from build123d import *

# Parameters (mm, degrees)
SKETCH_1_R          = 13
SKETCH_1_R_2        = 4
SKETCH_1_R_3        = 1.6
SKETCH_1_W          = 26
SKETCH_1_H          = 3
EXTRUDE_1_DEPTH     = 3
SKETCH_2_W          = 26
SKETCH_2_H          = 3
EXTRUDE_2_DEPTH     = 28
SKETCH_3_R          = 5
SKETCH_3_R_2        = 2
CUT_EXTRUDE_1_DEPTH = 44.0464865
EXTRUDE_3_DEPTH     = 3


with BuildPart() as part:
    # Sketch 1 → Extrude 1 (new body)
    # profile 1 of 3: a face of its own
    with BuildSketch(Plane(origin=(0, 0, 0), x_dir=(1, 0, 0), z_dir=(0, 1, 0))):
        Circle(SKETCH_1_R)
        with Locations(Location((0, 0, 0), (0, 0, 270))):
            Circle(SKETCH_1_R_2, mode=Mode.SUBTRACT)
        with Locations(Location((-8.5, 0, 0), (0, 0, 270))):
            Circle(SKETCH_1_R_3, mode=Mode.SUBTRACT)
        with Locations(Location((8.5, 0, 0), (0, 0, 270))):
            Circle(SKETCH_1_R_3, mode=Mode.SUBTRACT)
    # profile 2 of 3: a face of its own
    with BuildSketch(Plane(origin=(0, 0, 0), x_dir=(1, 0, 0), z_dir=(0, 1, 0))):
        with BuildLine():
            ThreePointArc((13, 0), (0, -13), (-13, 0))
            Line((-13, 0), (-13, -17))
            Line((-13, -17), (13, -17))
            Line((13, -17), (13, 0))
        make_face()
    # profile 3 of 3: a face of its own
    with BuildSketch(Plane(origin=(0, 0, 0), x_dir=(1, 0, 0), z_dir=(0, 1, 0))):
        with Locations((0, -18.5)):
            Rectangle(SKETCH_1_W, SKETCH_1_H)
    extrude(amount=EXTRUDE_1_DEPTH)

    # Sketch 2 → Extrude 2 (add)
    with BuildSketch(Plane.XZ):
        with Locations((0, 18.5)):
            Rectangle(SKETCH_2_W, SKETCH_2_H)
    extrude(amount=EXTRUDE_2_DEPTH)

    # Sketch 3 → Cut-Extrude 1 (cut, through all)
    with BuildSketch(Plane(origin=(0, 0, 17), x_dir=(-1, 0, 0), z_dir=(0, 0, -1))):
        with Locations((0, -14)):
            Circle(SKETCH_3_R)
        with Locations((8, -7)):
            Circle(SKETCH_3_R_2)
        with Locations((8, -21)):
            Circle(SKETCH_3_R_2)
        with Locations(Location((-8, -21, 0), (0, 0, 180))):
            Circle(SKETCH_3_R_2)
        with Locations(Location((-8, -7, 0), (0, 0, 180))):
            Circle(SKETCH_3_R_2)
    extrude(amount=-CUT_EXTRUDE_1_DEPTH, mode=Mode.SUBTRACT)

    # Sketch 3_4 → Extrude 3 (add)
    with BuildSketch(Plane(origin=(0, 0, 17), x_dir=(-1, 0, 0), z_dir=(0, 0, -1))):
        with BuildLine():
            ThreePointArc((13, -28), (12.472792206, -29.272792206), (11.2, -29.8))
            Line((11.2, -29.8), (-11.2, -29.8))
            ThreePointArc((-11.2, -29.8), (-12.472792206, -29.272792206), (-13, -28))
            Line((-13, -28), (13, -28))
        make_face()
    extrude(amount=-EXTRUDE_3_DEPTH)


solid = part.part
Model file for the job. Use its own axes, mm. A direction names the side the tool comes from. Give positions to 0.01 mm unless a question says otherwise; leave off trailing zeros. Loops run counter-clockwise (first coordinate to the right, second up) from the corner with the lowest first, then second, coordinate; pieces in that order, holes last.
1) Saw through at A-A (y = -7). Write the cut outline in (x, z), plus the area to 3 significant figures.
2) Flat gauge pins, fed straight in: pin 1 Ø3 at (x, z) = (-8, 5.5) entering from -Y; pin 2 Ø5 at (x, y) = (8, -7) entering from -Z; pin 3 Ø5 at (x, y) = (-2, -13) entering from -Z. Where does each tip first touch, or does it go through?
3) Pull direction Z, two halves, no side cores. Call faces 1 (the cylindrical face through (-10.06, 1.48, -0.35)), 2 (the flat face through (-3.1, -9.5, 20)), 3 (the flat face through (0, 0, 5)), 4 (the cylindrical face through (0, 1, -13)): +Z half, -Z half, draft (parallel to the pull), parting line (faces both ways), or undercut.
4) Wall check: line 1 (Y direction, x = -8, z = 18.7); line 2 (Z direction, x = 6, y = -20); line 3 (Y direction, x = 11.75, z = 6). Give the ranges that are in metal, low to high.
5) Saw through at C-C (y = -10.5). Write the cut outline in (x, z), plus the area to 3 significant figures.
6) Tool access for faces 5 (the flat face through (-6, -15, 17)), 6 (the flat face through (0, -29.8, 18)): list every direction of +Z, -Z, +X, -X, +Y, -Y with a clear straight run to the whole face (end or side of a thin tool).
7) Saw through at D-D (x = 8). Write the cut outline in (y, z), plus the area to 3 significant figures.
8) Saw through at B-B (x = 2.25). Write the cut outline in (y, z).
Answer block:
1. outline: (-13, 17) - (-10, 17) - (-10, 20) - (-13, 20) - close; (-6, 17) - (6, 17) - (6, 20) - (-6, 20) - close; (10, 17) - (13, 17) - (13, 20) - (10, 20) - close
1. area: 54.0 mm2
2. pin 1: stops at y = 0
2. pin 2: stops at z = 17
2. pin 3: passes through
3. face 1: undercut
3. face 2: +Z half
3. face 3: draft
3. face 4: -Z half
4. line 1: y = -29.8 to -23, -19 to -9, -5 to 3
4. line 2: z = 17 to 20
4. line 3: y = 0 to 3
5. outline: (-13, 17) - (-3.57, 17) - (-3.57, 20) - (-13, 20) - close; (3.57, 17) - (13, 17) - (13, 20) - (3.57, 20) - close
5. area: 56.6 mm2
6. face 5: -Z, +X, -X, -Y
6. face 6: +Z, -Z, +X, -X, -Y
7. outline: (-29.8, 17) - (-23, 17) - (-23, 20) - (-29.8, 20) - close; (-19, 17) - (-9, 17) - (-9, 20) - (-19, 20) - close; (-5, 17) - (0, 17) - (0, 1.52) - (3, 1.52) - (3, 20) - (-5, 20) - close; (0, -10.25) - (3, -10.25) - (3, -1.52) - (0, -1.52) - close
7. area: 147 mm2
8. outline: (-29.8, 17) - (-18.47, 17) - (-18.47, 20) - (-29.8, 20) - close; (-9.53, 17) - (0, 17) - (0, 3.31) - (3, 3.31) - (3, 20) - (-9.53, 20) - close; (0, -12.8) - (3, -12.8) - (3, -3.31) - (0, -3.31) - close
